```python
from build123d import *

# Parameters (mm, degrees)
EXTRUDE_1_DEPTH            = 90
HOLE_WIZARD_M81_AT_2_COUNT = 2
HOLE_WIZARD_M81_AT_2_PITCH = 63
HOLE_WIZARD_M81_AT_3_COUNT = 2
HOLE_WIZARD_M81_AT_3_PITCH = 93
HOLE_WIZARD_M81_AT_4_COUNT = 2
HOLE_WIZARD_M81_AT_4_PITCH = 156


with BuildPart() as part:
    # Эскиз1 → Бобышка-Вытянуть1 (new body, symmetric)
    with BuildSketch(Plane.XY):
        Polygon((5, 0), (-5, 0), (-5, -4.5), (-9.75, -4.5), (-9.75, -6.5), (-5, -10.5), (5, -10.5), (9.75, -6.5), (9.75, -4.5), (5, -4.5), align=None)
    extrude(amount=EXTRUDE_1_DEPTH, both=True)

    # Эскиз8 → Отверстие обработанное метчиком M81 (revolve, cut)
    with BuildSketch(Plane(origin=(0, 0, -78), x_dir=(0, 0, 1), z_dir=(1, 0, 0))):
        Polygon((0, 0), (0, 10.5), (4.025, 10.5), (3.4, 9.875), (3.4, 0.625), (4.025, 0), align=None)
    hole_wizard_m81 = revolve(axis=Axis((0, 6.35, -78), (0, -1, 0)), mode=Mode.SUBTRACT)

    # Отверстие обработанное метчиком M81 at 2: Отверстие обработанное метчиком M81 ×2
    with Locations(*[(0, 0, i * HOLE_WIZARD_M81_AT_2_PITCH) for i in range(1, HOLE_WIZARD_M81_AT_2_COUNT)]):
        add(hole_wizard_m81, mode=Mode.SUBTRACT)

    # Отверстие обработанное метчиком M81 at 3: Отверстие обработанное метчиком M81 ×2
    with Locations(*[(0, 0, i * HOLE_WIZARD_M81_AT_3_PITCH) for i in range(1, HOLE_WIZARD_M81_AT_3_COUNT)]):
        add(hole_wizard_m81, mode=Mode.SUBTRACT)

    # Отверстие обработанное метчиком M81 at 4: Отверстие обработанное метчиком M81 ×2
    with Locations(*[(0, 0, i * HOLE_WIZARD_M81_AT_4_PITCH) for i in range(1, HOLE_WIZARD_M81_AT_4_COUNT)]):
        add(hole_wizard_m81, mode=Mode.SUBTRACT)


solid = part.part
```
The model under review builds one solid part; all positions refer to its coordinate system, in mm. A direction names the side the tool comes from. Give positions to 0.01 mm unless a question says otherwise; leave off trailing zeros. Write each loop counter-clockwise with the first axis right and the second up, starting at its lowest first coordinate (ties: lowest second). Pieces come first, ordered by that corner, then holes. Notation, with made-up numbers: (89, -20) -> (112, -20) arc R5 cw to (112, -11) -> close; hole circle Ø6 at (19, -27). An arc over 180 degrees is marked (long way). Answer in a Markdown table with one row per item.
1) For L1, parallel to Z at x = 0, y = -3.5; L2, parallel to X at y = -4.75, z = -15; L3, parallel to X at y = -7, z = -15, list the stretches that pass through material, from the lowest coordinate up. Write a range as [from, to].
Worked answers:
| item | result |
|---|---|
| L1 | [-90, -81.4], [-74.6, -18.4], [-11.6, 11.6], [18.4, 74.6], [81.4, 90] |
| L2 | [-9.75, -3.4], [3.4, 9.75] |
| L3 | [-9.16, -3.4], [3.4, 9.16] |
2) Add section A-A on y = -2.75. State the section outline as (x, z) points.
Worked answers:
| item | result |
|---|---|
| outline | (-5, -90) -> (5, -90) -> (5, 90) -> (-5, 90) -> close; hole circle Ø6.8 at (0, -78); hole circle Ø6.8 at (0, -15); hole circle Ø6.8 at (0, 15); hole circle Ø6.8 at (0, 78) |
3) Add section C-C on z = -55.5. State the section outline as (x, y) points, plus the area to 3 significant figures.
Worked answers:
| item | result |
|---|---|
| outline | (-9.75, -6.5) -> (-5, -10.5) -> (5, -10.5) -> (9.75, -6.5) -> (9.75, -4.5) -> (5, -4.5) -> (5, 0) -> (-5, 0) -> (-5, -4.5) -> (-9.75, -4.5) -> close |
| area | 143 mm² |
4) Mouldability with a two-part tool opening along Z and no side actions: class faces 4 (the flat face through (0, -5, -90)), 5 (the flat face through (0, -5, 90)), 6 (the cylindrical face through (-0.1, -5.2, 11.6)) as +Z half, -Z half, draft (parallel to the pull), parting line (faces both ways), or undercut.
Worked answers:
| item | result |
|---|---|
| face 4 | -Z half |
| face 5 | +Z half |
| face 6 | undercut |
5) Clearance check with flat-ended pins moving along their axes: P1, Ø5, axis at y = -9.5, z = 7.5, coming from the +X side; P2, Ø1.5, axis at y = -8, z = -60.5, coming from the +X side; P3, Ø2.5, axis at x = -7.5, z = 40.5, coming from the +Y side. State where each tip first meets the part, or that it passes through.
Worked answers:
| item | result |
|---|---|
| P1 | x = 9.16 |
| P2 | x = 8.86 |
| P3 | y = -4.5 |
6) Tool access review of faces 1 (the flat face through (5, -2, 1)), 2 (the flat face through (-5, -2, 1)), 3 (the cylindrical face through (-0.1, -5.2, -81.4)): name each direction out of +Z, -Z, +X, -X, +Y, -Y from which nothing blocks a thin tool from reaching the whole face with its end or side.
Worked answers:
| item | result |
|---|---|
| face 1 | +Z, -Z, +X, +Y |
| face 2 | +Z, -Z, -X, +Y |
| face 3 | +Y, -Y |
7) Add section B-B on z = 78. State the section outline as (x, y) points (3 decimals), plus the area to 3 significant figures.
Worked answers:
| item | result |
|---|---|
| outline | (-9.75, -6.5) -> (-5, -10.5) -> (-4.025, -10.5) -> (-3.4, -9.875) -> (-3.4, -0.625) -> (-4.025, 0) -> (-5, 0) -> (-5, -4.5) -> (-9.75, -4.5) -> close; (3.4, -9.875) -> (4.025, -10.5) -> (5, -10.5) -> (9.75, -6.5) -> (9.75, -4.5) -> (5, -4.5) -> (5, 0) -> (4.025, 0) -> (3.4, -0.625) -> close |
| area | 70.8 mm² |
